Check sheet for the drawn part. Datum: minimum x, y, z corner. Units: mm. Give positions to 0.01 mm unless a question says otherwise; leave off trailing zeros. Write each loop counter-clockwise with the first axis right and the second up, starting at its lowest first coordinate (ties: lowest second). Pieces come first, ordered by that corner, then holes. Notation, with made-up numbers: (2.25, 48.5) - (38.25, 48.5) arc R25 cw to (38.25, 76.5) - close; hole circle Ø3 at (-13.75, -15.5). An arc over 180 degrees is marked (long way). Answer as a JSON object with one key per item and string values. Group by question number.
Item 1: Sectioned sample at B-B, the plane z = 16. Record the boundary of the cut face in (x, y) (1 decimal).
Item 2: Sectioned sample at A-A, the plane x = 19.05. Count the separate pieces of the cut face and the enclosed holes in it.
Item 3: Go/stop test with a flat-tipped pin: pin 1 (2.5 mm diameter, centred on x = 19.05, z = 3.175, fed in from +Y). Record where the tip stops, or that it passes through.
Item 4: Scan lines: line 1 along X through (y, z) = (2.75, 41.5) (1 decimal); line 2 along X through (y, z) = (4.25, 66) (1 decimal); line 3 along Z through (x, y) = (24.5, 3). Record each from-to range of solid material in increasing order. Write a range as [from, to].
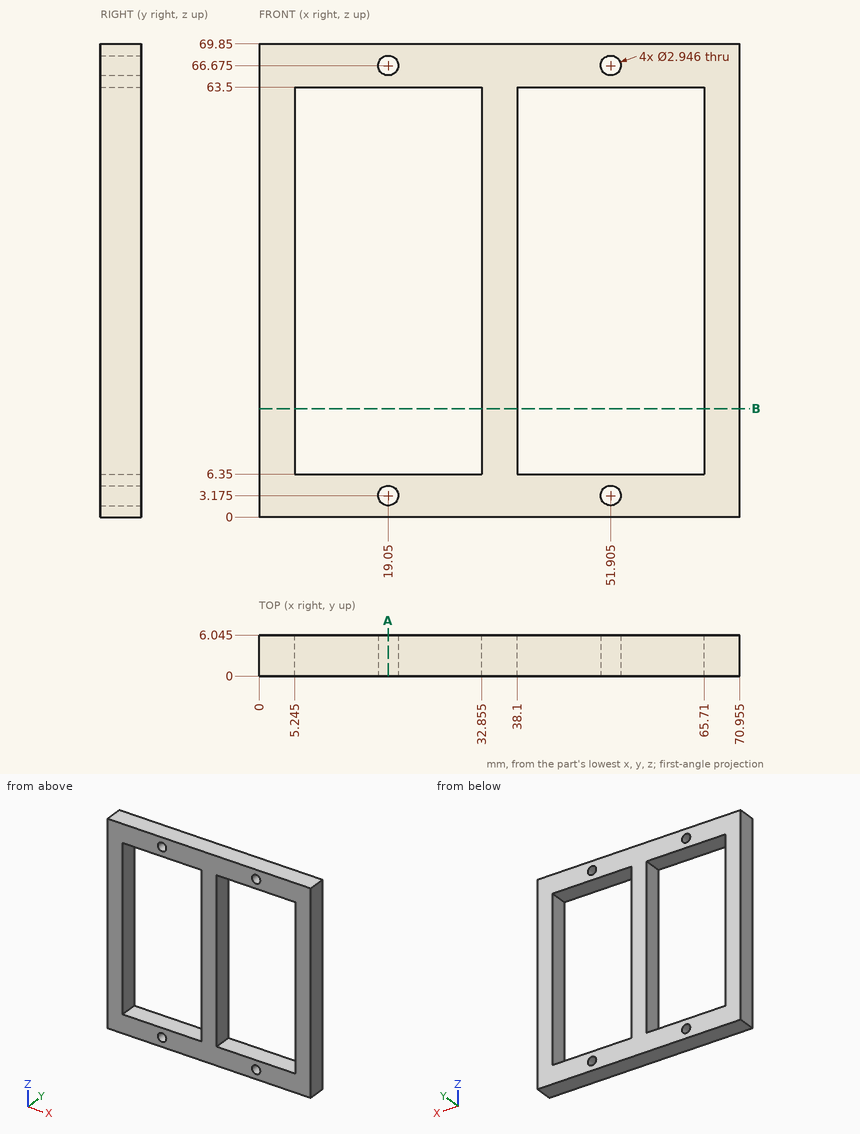
Geometry check:
{
 "1": {"outline": "(0, 0) - (5.2, 0) - (5.2, 6) - (0, 6) - close; (32.9, 0) - (38.1, 0) - (38.1, 6) - (32.9, 6) - close; (65.7, 0) - (71, 0) - (71, 6) - (65.7, 6) - close"},
 "2": {"separate pieces": "4", "enclosed holes": "0"},
 "3": {"pin 1": "through"},
 "4": {"line 1": "[0, 5.2], [32.9, 38.1], [65.7, 71]", "line 2": "[0, 17.7], [20.4, 50.6], [53.2, 71]", "line 3": "[0, 6.35], [63.5, 69.85]"}
}
